CAD build for the part. Positions are in the model's coordinates, mm. A direction names the side the tool comes from. Give positions to 0.01 mm unless a question says otherwise; leave off trailing zeros. Order: outer loops, then holes, each group sorted by start corner. A loop starts at its lowest first (then second) coordinate and runs counter-clockwise, first axis right, second up. Notation, with made-up numbers: M -4,61 L 26,61 A23 cw 26,69 Z; hole C -27.75,75.25 d5. An arc over 180 degrees is marked long. Put each result on its own line as item: value. Start each with the question number.
1) Cut at C-C (y = 2.75). Write the cut outline in (x, z), and give its area (3 significant figures).
2) Two-plate mould, pull along X, no slides. Class faces 5 (the face through (0, 1, 7.5)), 6 (the face through (13, 8, 1)), 7 (the face through (0, 14, 5.5)), 8 (the face through (-15, 7, 0)): released by +X, released by -X, zero draft, split by the parting line, or undercut.
3) Pin check, flat tips, straight feed: pin 1 (3.5 mm diameter, centred on x = 4, y = 5.5, fed in from +Z); pin 2 (4 mm diameter, centred on x = 5.5, y = 12, fed in from -Z); pin 3 (1 mm diameter, centred on x = 4.5, y = 13.5, fed in from -Z). Stop position of each tip, or through.
4) Tool access for faces 1 (the face through (0, 2, 7)), 2 (the face through (0, 6, -5.5)), 3 (the face through (0, 13, 7)), 4 (the face through (0, 0, 7)): list every direction of +Z, -Z, +X, -X, +Y, -Y with a clear straight run to the whole face (end or side of a thin tool).
5) Cut at B-B (x = 5.5). Write the cut outline in (y, z).
6) Cut at D-D (z = -2.5). Write the cut outline in (x, y), and give its area (3 significant figures).
7) Drill centre lines: line 1 (X direction, y = 6.5, z = -2.5); line 2 (Y direction, x = -11.25, z = 6.75); line 3 (Z direction, x = 10.75, y = 1.5). Where is each one in solid material? Low to high. Write a range as [from, to].
8) Cut at A-A (z = 3). Write the cut outline in (x, y), and give its area (3 significant figures).
```python
from build123d import *

# Parameters (mm, degrees)
SKETCH12_W              = 30
SKETCH12_H              = 15
BOSS_EXTRUDE4_DEPTH     = 15
FILLET1_R               = 10
CUT_EXTRUDE8_DEPTH      = 23.5
CUT_EXTRUDE8_DEPTH_BACK = 23.5
SKETCH13_W              = 26
SKETCH13_H              = 11
SKETCH14_W              = 26
SKETCH14_H              = 11
CUT_EXTRUDE9_DEPTH      = 10


with BuildPart() as part:
    # Sketch12 → Boss-Extrude4 (new body)
    with BuildSketch(Plane(origin=(0, 0, 0), x_dir=(1, 0, 0), z_dir=(0, 1, 0))):
        Rectangle(SKETCH12_W, SKETCH12_H)
    extrude(amount=BOSS_EXTRUDE4_DEPTH)

    # Fillet1
    fillet1_edges = [part.edges().sort_by_distance(p)[0] for p in [
        (0, 15, -7.5),
    ]]
    fillet(fillet1_edges, radius=FILLET1_R)

    # Sketch13 → Cut-Extrude8 (cut, two sides: drawn at the far end of the back side and taken through both)
    with BuildSketch(Plane.XZ.offset(-CUT_EXTRUDE8_DEPTH_BACK)):
        Rectangle(SKETCH13_W, SKETCH13_H)
    extrude(amount=CUT_EXTRUDE8_DEPTH + CUT_EXTRUDE8_DEPTH_BACK, mode=Mode.SUBTRACT)

    # Sketch14 → Cut-Extrude9 (cut)
    with BuildSketch(Plane.XY.offset(7.5)):
        with Locations((0, 7.5)):
            Rectangle(SKETCH14_W, SKETCH14_H)
    extrude(amount=-CUT_EXTRUDE9_DEPTH, mode=Mode.SUBTRACT)


solid = part.part
```
Solution:
1. outline: M -15,-7.5 L 15,-7.5 L 15,7.5 L 13,7.5 L 13,-5.5 L -13,-5.5 L -13,7.5 L -15,7.5 Z
1. area: 112 mm²
2. face 5: zero draft
2. face 6: undercut
2. face 7: undercut
2. face 8: released by -X
3. pin 1: z = -5.5
3. pin 2: z = -6.16
3. pin 3: z = 5.5
4. face 1: +Z
4. face 2: +Y, -Y
4. face 3: +Z, -Z
4. face 4: +Z, -Z, +X, -X, -Y
5. outline: M 0,-7.5 L 5,-7.5 A10 ccw 11,-5.5 L 0,-5.5 Z; M 0,5.5 L 2,5.5 L 2,7.5 L 0,7.5 Z; M 13,5.5 L 15,5.5 L 15,7.5 L 13,7.5 Z
6. outline: M -15,0 L -13,0 L -13,13.66 L -15,13.66 Z; M 13,0 L 15,0 L 15,13.66 L 13,13.66 Z
6. area: 54.6 mm²
7. line 1: [-15, -13], [13, 15]
7. line 2: [0, 2], [13, 15]
7. line 3: [-7.5, -5.5], [5.5, 7.5]
8. outline: M -15,0 L -13,0 L -13,15 L -15,15 Z; M 13,0 L 15,0 L 15,15 L 13,15 Z
8. area: 60.0 mm²
